Verification items for the finished model (mm, model axes). A direction names the side the tool comes from. Coordinates: 2 decimals unless noted, no trailing zeros. Loops run counter-clockwise (first coordinate to the right, second up) from the corner with the lowest first, then second, coordinate; pieces in that order, holes last. Notation, with made-up numbers: (57.25, 60) - (92.25, 60) arc R20 cw to (92.25, 92) - close; hole circle Ø3 at (50, -30). An arc over 180 degrees is marked (long way). One line per item, written item: value. Start each with the question number.
(1) Section check B-B (z = -16). Count the separate pieces of the cut face and the enclosed holes in it, plus the area to 3 significant figures.
(2) Section check A-A (y = -41). Record the boundary of the cut face in (x, z), plus the area to 3 significant figures.
(3) Set-up check for faces 5 (the face through (-4, -32, 6)), 6 (the face through (-10, -45, -5.2)), 7 (the face through (12.32, -37, -7)), 8 (the face through (9.304, -45.015, -5.808)): record each of +Z, -Z, +X, -X, +Y, -Y from which the full face is reachable in a straight line by a thin tool's end or side.
(4) Thickness scan on probe 1 along X at (y, z) = (-40.5, -3.5); probe 2 along X at (y, z) = (-11, -16); probe 3 along Z at (x, y) = (-16, -6). Record the ranges inside material, lowest first. Write a range as [from, to].
(5) Draft check along Y on faces 1 (the face through (-10.238, -43.358, -5.808)), 2 (the face through (11.093, -43.044, -7.061)), 3 (the face through (-3.34, -31.73, -18.78)), 4 (the face through (15.686, -8.114, 14.584)). Enter one of: +Y half, -Y half, draft (parallel to the pull), parting line (faces both ways), or undercut.
(6) Gauge pin test, flat ends, axial feed: P1, Ø3, axis at y = -15, z = -9, coming from the -X side; P2, Ø1, axis at x = -10, y = -45.5, coming from the +Z side; P3, Ø1, axis at x = -10, y = -45, coming from the -Z side. Record the tip position at first contact, or that the pin passes through.
```python
from build123d import *

# Parameters (mm, degrees)
SKETCH_W        = 40
SKETCH_H        = 40
SKETCH001_W     = 40
SKETCH001_H     = 40
SKETCH002_W     = 28.2
SKETCH002_H     = 28
SKETCH015_W     = 24.64
SKETCH015_H     = 26
SKETCH003_W     = 24.64
SKETCH003_H     = 26
PAD001_DEPTH    = 11.10001
PAD_DEPTH       = 26
SKETCH013_W     = 24.64
SKETCH013_H     = 24.64
SKETCH009_W     = 22.2
SKETCH009_H     = 23.56
SKETCH017_W     = 22.2
SKETCH017_H     = 23.56
POCKET001_DEPTH = 11.10001
SKETCH010_R     = 11.1
POCKET_DEPTH    = 40
PAD002_DEPTH    = 1.2
SKETCH011_R     = 1.45
POCKET002_DEPTH = 46.864698
CHAMFER_SIZE    = 1.4


with BuildPart() as part:
    # Sketch → AdditiveLoft section 0
    with BuildSketch(Plane.XZ):
        Rectangle(SKETCH_W, SKETCH_H)
    # Sketch001 → AdditiveLoft section 1
    with BuildSketch(Plane.XZ.offset(6)):
        Rectangle(SKETCH001_W, SKETCH001_H)
    # Sketch002 → AdditiveLoft section 2
    with BuildSketch(Plane.XZ.offset(26)):
        with Locations((0, -6)):
            Rectangle(SKETCH002_W, SKETCH002_H)
    # Sketch015 → AdditiveLoft section 3
    with BuildSketch(Plane.XZ.offset(31.55)):
        with Locations((0, -7)):
            Rectangle(SKETCH015_W, SKETCH015_H)
    loft()

    # Sketch003 → Pad001 (new body)
    with BuildSketch(Plane.XZ.offset(31.55)):
        with Locations((0, -7)):
            Rectangle(SKETCH003_W, SKETCH003_H)
    extrude(amount=PAD001_DEPTH)

    # Sketch004 → Pad (join)
    with BuildSketch(Plane.XY.offset(-20)):
        with BuildLine():
            ThreePointArc((11.577013, -46.863698), (0, -30.33001), (-11.577013, -46.863698))
            Line((-11.577013, -46.863698), (11.577013, -46.863698))
        make_face()
    extrude(amount=PAD_DEPTH)

    # Sketch006 → SubtractiveLoft section 0
    with BuildSketch(Plane.XZ):
        with BuildLine():
            ThreePointArc((15.809634, 11.070025), (0, 19.3), (-15.809634, 11.070025))
            ThreePointArc((-15.809634, 11.070025), (-19.3, 0), (-15.809634, -11.070025))
            ThreePointArc((-15.809634, -11.070025), (0, -19.3), (15.809634, -11.070025))
            ThreePointArc((15.809634, -11.070025), (19.3, 0), (15.809634, 11.070025))
        make_face()
    # Sketch005 → SubtractiveLoft section 1
    with BuildSketch(Plane.XZ.offset(6)):
        with BuildLine():
            ThreePointArc((14.699251, 10.690132), (0, 17.939), (-14.699251, 10.690132))
            ThreePointArc((-14.699251, 10.690132), (-18.528, -0.589), (-14.699251, -11.868132))
            ThreePointArc((-14.699251, -11.868132), (0, -19.117), (14.699251, -11.868132))
            ThreePointArc((14.699251, -11.868132), (18.528, -0.589), (14.699251, 10.690132))
        make_face()
    # Sketch013 → SubtractiveLoft section 2
    with BuildSketch(Plane.XZ.offset(26)):
        with Locations((0, -6.46)):
            Rectangle(SKETCH013_W, SKETCH013_H)
    # Sketch009 → SubtractiveLoft section 3
    with BuildSketch(Plane.XZ.offset(31.55)):
        with Locations((0, -7)):
            Rectangle(SKETCH009_W, SKETCH009_H)
    loft(mode=Mode.SUBTRACT)

    # Sketch017 → Pocket001 (cut)
    with BuildSketch(Plane.XZ.offset(31.55)):
        with Locations((0, -7)):
            Rectangle(SKETCH017_W, SKETCH017_H)
    extrude(amount=POCKET001_DEPTH, mode=Mode.SUBTRACT)

    # Sketch010 → Pocket (cut)
    with BuildSketch(Plane.XY.offset(-20)):
        with Locations((0, -42.65001)):
            Circle(SKETCH010_R)
    extrude(amount=POCKET_DEPTH, mode=Mode.SUBTRACT)

    # Sketch012 → Pad002 (join)
    with BuildSketch(Plane.XY.offset(-6.4)):
        with BuildLine():
            ThreePointArc((-11.2, -42.65001), (-11.029847, -44.59487), (-10.524557, -46.480636))
            Line((-10.524557, -46.480636), (-9.021049, -45.933403))
            ThreePointArc((-9.6, -42.65001), (-9.454154, -44.317033), (-9.021049, -45.933403))
            Line((-11.2, -42.65001), (-9.6, -42.65001))
        make_face()
        with BuildLine():
            Line((9.021049, -45.933403), (10.524557, -46.480636))
            ThreePointArc((10.524557, -46.480636), (11.029847, -44.59487), (11.2, -42.65001))
            Line((9.6, -42.65001), (11.2, -42.65001))
            ThreePointArc((9.021049, -45.933403), (9.454154, -44.317033), (9.6, -42.65001))
        make_face()
    extrude(amount=PAD002_DEPTH)

    # Sketch011 → Pocket002 (cut, through all)
    with BuildSketch(Plane.XZ):
        with Locations((-16, 16)):
            Circle(SKETCH011_R)
        with Locations((16, 16)):
            Circle(SKETCH011_R)
        with Locations((16, -16)):
            Circle(SKETCH011_R)
        with Locations((-16, -16)):
            Circle(SKETCH011_R)
    extrude(amount=POCKET002_DEPTH, mode=Mode.SUBTRACT)

    # Chamfer
    chamfer_edges = [part.edges().sort_by_distance(p)[0] for p in [
        (9.6, -42.65001, -5.8),
        (-9.6, -42.65001, -5.8),
    ]]
    chamfer(chamfer_edges, length=CHAMFER_SIZE)


solid = part.part
```
Responses:
1. separate pieces: 4
1. enclosed holes: 0
1. area: 266 mm²
2. outline: (-12.32, -20) - (-10.98, -20) - (-10.98, -18.78) - (-11.1, -18.78) - (-11.1, 4.78) - (-10.98, 4.78) - (-10.98, 6) - (-12.32, 6) - close; (10.98, -20) - (12.32, -20) - (12.32, 6) - (10.98, 6) - (10.98, 4.78) - (11.1, 4.78) - (11.1, -18.78) - (10.98, -18.78) - close
2. area: 64.0 mm²
3. face 5: +Z, +X, -X, -Y
3. face 6: +Z, +Y
3. face 7: +Z, -Z, +X, -Y
3. face 8: +Z, -Z, +Y
4. probe 1: x = [-12.32, -11.1], [11.1, 12.32]
4. probe 2: x = [-19.2, -17.45], [-14.55, -10.82], [10.82, 14.55], [17.45, 19.2]
4. probe 3: z = [-20, -17.45], [-14.55, -9.93], [8.75, 14.55], [17.45, 20]
5. face 1: +Y half
5. face 2: undercut
5. face 3: undercut
5. face 4: draft
6. P1: stops at x = -18.56
6. P2: stops at z = -5.2
6. P3: stops at z = -6.4
